Geometry: see drawing. Coordinates: mm, zero at the bounding-box minimum. Give positions to 0.01 mm unless a question says otherwise; leave off trailing zeros. Order: outer loops, then holes, each group sorted by start corner. A loop starts at its lowest first (then second) coordinate and runs counter-clockwise, first axis right, second up. Notation, with made-up numbers: (-25.5, 84.5) - (25.5, 84.5) arc R19 cw to (25.5, 112.5) - close; hole circle Ø6 at (80.25, 82.25). An arc over 180 degrees is marked (long way). Put each result on its own line as item: value. Start each with the question number.
1. Section B-B on x = 28.5. Return the cut outline in (y, z), plus the area to 3 significant figures.
2. Section D-D on z = 28.5. Return the cut outline in (x, y), plus the area to 3 significant figures.
3. First-contact query: P1, Ø14.5, axis at x = 54.5, z = 17.5, coming from the -Y side; P2, Ø1.5, axis at y = 0.5, z = 3.5, coming from the -X side. Flat tips, straight axial feed; report the tip coordinate or a pass-through.
4. Section C-C on y = 1.35. Count the separate pieces of the cut face and the enclosed holes in it, plus the area to 3 significant figures.
5. Ray query, line 1 along Z through (x, y) = (69.25, 1.2); line 2 along Z through (x, y) = (8.75, 1.6); line 3 along Z through (x, y) = (28.5, 1.45). Return the intervals inside material, ascending. Write a range as from..to.
6. Section A-A on x = 8.75. Return the cut outline in (y, z), plus the area to 3 significant figures.
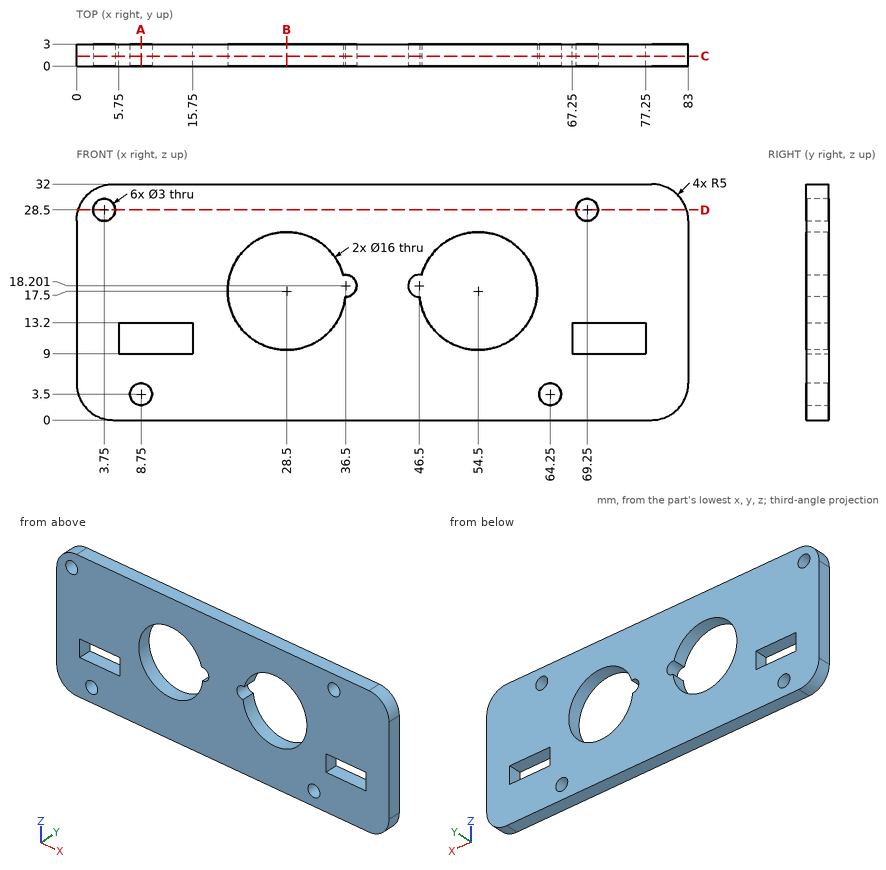
Resolved:
1. outline: (0, 0) - (3, 0) - (3, 9.5) - (0, 9.5) - close; (0, 25.5) - (3, 25.5) - (3, 32) - (0, 32) - close
1. area: 48.0 mm^2
2. outline: (0.23, 0) - (2.25, 0) - (2.25, 3) - (0.23, 3) - close; (5.25, 0) - (67.75, 0) - (67.75, 3) - (5.25, 3) - close; (70.75, 0) - (82.77, 0) - (82.77, 3) - (70.75, 3) - close
2. area: 230 mm^2
3. P1: through
3. P2: x = 0.06
4. separate pieces: 1
4. enclosed holes: 8
4. area: 2,110 mm^2
5. line 1: 0..9, 13.2..27, 30..32
5. line 2: 0..2, 5..9, 13.2..32
5. line 3: 0..9.5, 25.5..32
6. outline: (0, 0) - (3, 0) - (3, 2) - (0, 2) - close; (0, 5) - (3, 5) - (3, 9) - (0, 9) - close; (0, 13.2) - (3, 13.2) - (3, 32) - (0, 32) - close
6. area: 74.4 mm^2
